from build123d import *

# Parameters (mm, degrees)
ESBO_O1_R                     = 1.55
RESSALTO_EXTRUS_O1_DEPTH      = 1.6
ESBO_O2_W                     = 10
ESBO_O2_H                     = 13
RESSALTO_EXTRUS_O2_DEPTH      = 7
RESSALTO_EXTRUS_O3_DEPTH      = 1
RESSALTO_EXTRUS_O3_DEPTH_BACK = 7


with BuildPart() as part:
    # Esboço1 → Ressalto-extrusão1 (new body)
    with BuildSketch(Plane.XY):
        with BuildLine():
            Line((-30.175, 18.835), (30.175, 18.835))
            ThreePointArc((30.175, 18.835), (32.313998013, 17.948998013), (33.2, 15.81))
            Line((33.2, 15.81), (33.2, -15.81))
            ThreePointArc((33.2, -15.81), (32.313998013, -17.948998013), (30.175, -18.835))
            Line((30.175, -18.835), (-30.175, -18.835))
            ThreePointArc((-30.175, -18.835), (-32.313998013, -17.948998013), (-33.2, -15.81))
            Line((-33.2, -15.81), (-33.2, 15.81))
            ThreePointArc((-33.2, 15.81), (-32.313998013, 17.948998013), (-30.175, 18.835))
        make_face()
        with Locations((-30.175, 15.81)):
            Circle(ESBO_O1_R, mode=Mode.SUBTRACT)
        with Locations((-30.175, -15.81)):
            Circle(ESBO_O1_R, mode=Mode.SUBTRACT)
        with Locations((17.455, 15.81)):
            Circle(ESBO_O1_R, mode=Mode.SUBTRACT)
        with Locations((17.455, -15.81)):
            Circle(ESBO_O1_R, mode=Mode.SUBTRACT)
    extrude(amount=RESSALTO_EXTRUS_O1_DEPTH)

    # Esboço2 → Ressalto-extrusão2 (add)
    with BuildSketch(Plane.XY.offset(1.6)):
        with Locations((29.2, 9.31)):
            Rectangle(ESBO_O2_W, ESBO_O2_H)
        with Locations((29.2, -9.31)):
            Rectangle(ESBO_O2_W, ESBO_O2_H)
    extrude(amount=RESSALTO_EXTRUS_O2_DEPTH)

    # Esboço3 → Ressalto-extrusão3 (add, two sides)
    with BuildSketch(Plane.ZY.offset(33.2)) as ressalto_extrus_o3_sk:
        with BuildLine():
            Line((5.1, 2.75), (5.1, -2.75))
            ThreePointArc((5.1, -2.75), (3.35, -4.5), (1.6, -2.75))
            Line((1.6, -2.75), (1.6, 2.75))
            ThreePointArc((1.6, 2.75), (3.35, 4.5), (5.1, 2.75))
        make_face()
    extrude(amount=RESSALTO_EXTRUS_O3_DEPTH)
    extrude(ressalto_extrus_o3_sk.sketch, amount=-RESSALTO_EXTRUS_O3_DEPTH_BACK)


solid = part.part
Verification items for the finished model (mm, model axes). A direction names the side the tool comes from. Round coordinates to 2 decimals unless told otherwise and drop trailing zeros. Loops run counter-clockwise (first coordinate to the right, second up) from the corner with the lowest first, then second, coordinate; pieces in that order, holes last. Notation, with made-up numbers: (82, 21.5) - (91, 21.5) arc R32 ccw to (91, 51.5) - close; hole circle Ø5 at (13.5, 9.25). An arc over 180 degrees is marked (long way). Answer in a Markdown table with one row per item. Add a question column.
Q1. Section check A-A on z = 3.35. Enter the section's corners in (x, y), plus the area to 3 significant figures.
Q2. Material ranges on line 1 (Y direction, x = 29, z = 2.75); line 2 (X direction, y = 14.5, z = 1.75); line 3 (Z direction, x = -7, y = 11.5), recorded low to high.
Q3. Section check C-C on y = 5.5. Enter the section's corners in (x, z), plus the area to 3 significant figures.
Q4. Release check for a two-part mould opening along Y. For faces 5 (the face through (29, 15.81, 5)), 6 (the face through (33.2, 0, 1)), 7 (the face through (29, -2.81, 5)) record: pulls with the +Y half, pulls with the -Y half, needs draft (parallel to the pull), parting line crosses it, or undercut.
Q5. Tool access check on faces 1 (the face through (-31.724, -15.742, 0.789)), 2 (the face through (29, -15.81, 5)), 3 (the face through (-26.2, 0, 3)), 4 (the face through (29, 2.81, 5)). Record the directions out of +Z, -Z, +X, -X, +Y, -Y that give a thin tool (end or side, any length) a straight path to the whole face; none if there is none.
Q6. Section check D-D on x = -1. Enter the section's corners in (y, z) (3 decimals).
Q7. Gauge pin test, flat ends, axial feed: pin 1 (3.5 mm diameter, centred on x = 29.5, z = 3.5, fed in from +Y); pin 2 (1.1 mm diameter, centred on x = -34, y = -0.5, fed in from -Z); pin 3 (5 mm diameter, centred on x = 3.5, y = -12.5, fed in from -Z); pin 4 (3.5 mm diameter, centred on y = 8.5, z = 5.5, fed in from -X). Record the tip position at first contact, or that the pin passes through.
Q8. Section check B-B on z = 7.25. Enter the section's corners in (x, y).
Found:
| question | item | result |
|---|---|---|
| 1 | outline | (-34.2, -4.5) - (-26.2, -4.5) - (-26.2, 4.5) - (-34.2, 4.5) - close; (24.2, -15.81) - (34.2, -15.81) - (34.2, -2.81) - (24.2, -2.81) - close; (24.2, 2.81) - (34.2, 2.81) - (34.2, 15.81) - (24.2, 15.81) - close |
| 1 | area | 332 mm² |
| 2 | line 1 | y = -15.81 to -2.81, 2.81 to 15.81 |
| 2 | line 2 | x = 24.2 to 34.2 |
| 2 | line 3 | z = 0 to 1.6 |
| 3 | outline | (-33.2, 0) - (33.2, 0) - (33.2, 1.6) - (34.2, 1.6) - (34.2, 8.6) - (24.2, 8.6) - (24.2, 1.6) - (-33.2, 1.6) - close |
| 3 | area | 176 mm² |
| 4 | face 5 | pulls with the +Y half |
| 4 | face 6 | needs draft |
| 4 | face 7 | undercut |
| 5 | face 1 | +Z, -Z |
| 5 | face 2 | +Z, +X, -X, -Y |
| 5 | face 3 | +Z, +Y, -Y |
| 5 | face 4 | +Z, +X |
| 6 | outline | (-18.835, 0) - (18.835, 0) - (18.835, 1.6) - (-18.835, 1.6) - close |
| 7 | pin 1 | stops at y = 15.81 |
| 7 | pin 2 | stops at z = 1.6 |
| 7 | pin 3 | stops at z = 0 |
| 7 | pin 4 | stops at x = 24.2 |
| 8 | outline | (24.2, -15.81) - (34.2, -15.81) - (34.2, -2.81) - (24.2, -2.81) - close; (24.2, 2.81) - (34.2, 2.81) - (34.2, 15.81) - (24.2, 15.81) - close |
